Build history of the part. All positions in model axes, mm. Give positions to 0.01 mm unless a question says otherwise; leave off trailing zeros. Order: outer loops, then holes, each group sorted by start corner. A loop starts at its lowest first (then second) coordinate and runs counter-clockwise, first axis right, second up. Notation, with made-up numbers: (39.25, 38) - (94.25, 38) arc R7 ccw to (94.25, 45) - close; hole circle Ø7 at (33, 66.5). An arc over 180 degrees is marked (long way). Answer in a Markdown table with one row per item.
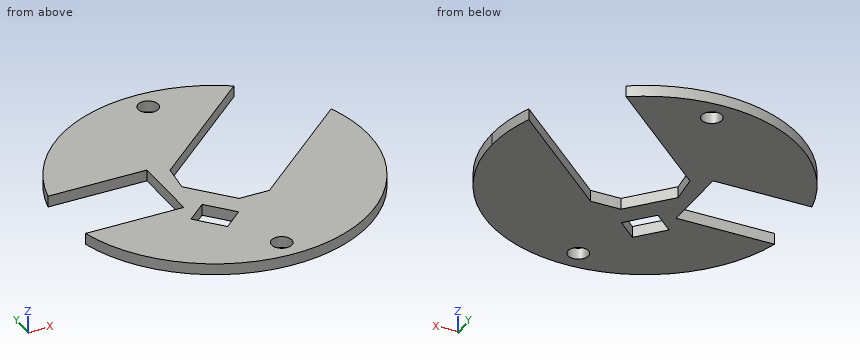
```python
from build123d import *

# Parameters (mm, degrees)
SKETCH1_R           = 1.4224
BOSS_EXTRUDE1_DEPTH = 1.5875


with BuildPart() as part:
    # Sketch1 → Boss-Extrude1 (new body)
    with BuildSketch(Plane.XY):
        with BuildLine():
            Line((-5.027565338, -0.720652536), (-4.515281158, 3.5306))
            Line((-4.515281158, 3.5306), (11.876076152, 18.030166811))
            ThreePointArc((11.876076152, 18.030166811), (-8.013144755, 20.047882959), (-21.031997569, 4.8768))
            Line((-21.031997569, 4.8768), (-7.084965338, 4.8768))
            Line((-7.084965338, 4.8768), (-7.084965338, -5.2832))
            Line((-7.084965338, -5.2832), (-20.933606898, -5.2832))
            ThreePointArc((-20.933606898, -5.2832), (2.661909754, -21.425273311), (21.59, 0))
            ThreePointArc((21.59, 0), (21.246782402, 3.834362733), (20.228041911, 7.546815251))
            Line((20.228041911, 7.546815251), (4.353635591, -6.495463901))
            Line((4.353635591, -6.495463901), (0.080752517, -6.495463901))
            Line((0.080752517, -6.495463901), (-5.027565338, -0.720652536))
        make_face()
        with Locations((0, -18.415)):
            Circle(SKETCH1_R, mode=Mode.SUBTRACT)
        Polygon((-7.562063797, -8.206208525), (-4.708345419, -5.681848919), (-1.443506996, -9.372658021), (-4.297225374, -11.897017627), align=None, mode=Mode.SUBTRACT)
        with Locations((0, 18.415)):
            Circle(SKETCH1_R, mode=Mode.SUBTRACT)
    extrude(amount=BOSS_EXTRUDE1_DEPTH)


solid = part.part
```
1. Cut at A-A on x = -14. Write the cut outline in (y, z), and give its area (3 significant figures).
Check result:
| item | result |
|---|---|
| outline | (-16.44, 0) - (-5.28, 0) - (-5.28, 1.59) - (-16.44, 1.59) - close; (4.88, 0) - (16.44, 0) - (16.44, 1.59) - (4.88, 1.59) - close |
| area | 36.1 mm² |
2. Probe line 1 (Y direction, x = 0, z = 0.5); line 2 (X direction, y = -4.5, z = 0.2); line 3 (Y direction, x = -9.5, z = 1.5). List the from-to ranges inside material, lowest first.
Check result:
| item | result |
|---|---|
| line 1 | y = -21.59 to -19.84, -16.99 to -6.4, 7.52 to 16.99, 19.84 to 21.59 |
| line 2 | x = -7.08 to -1.68, 6.61 to 21.12 |
| line 3 | y = -19.39 to -5.28, 4.88 to 19.39 |
3. Drop flat-ended pins along their axis: P1, Ø0.5, axis at x = 3, z = 0.5, coming from the +Y side; P2, Ø0.5, axis at x = -15.5, z = 0.5, coming from the +Y side. Give the stop position or say it passes through.
Check result:
| item | result |
|---|---|
| P1 | stops at y = 21.41 |
| P2 | stops at y = 15.28 |
4. Cut at B-B on y = 6. Write the cut outline in (x, z), and give its area (3 significant figures).
Check result:
| item | result |
|---|---|
| outline | (-20.74, 0) - (-1.72, 0) - (-1.72, 1.59) - (-20.74, 1.59) - close; (18.48, 0) - (20.74, 0) - (20.74, 1.59) - (18.48, 1.59) - close |
| area | 33.8 mm² |
